```python
from build123d import *

# Parameters (mm, degrees)
F1_DEPTH = 20
F4_W     = 74.543075636
F4_H     = 79.5415919274
F5_DEPTH = 23.0950107676
F7_W     = 62.1554479003
F7_H     = 78.672291711
F8_DEPTH = 25


with BuildPart() as f1:
    # F0 (on Right) → F1 (new body, symmetric)
    with BuildSketch(Plane.YZ):
        Polygon((0, 20), (0, 0), (40, 0), (40, 40), align=None)
    extrude(amount=F1_DEPTH, both=True)

    # F4 (on 3pt) → F5 (cut, through all)
    with BuildSketch(Plane(origin=(6.6666666667, -6.6666666667, 6.6666666667), x_dir=(0.8164965809, 0.4082482905, -0.4082482905), z_dir=(0.5773502692, -0.5773502692, 0.5773502692))):
        with Locations((13.7506006286, 22.7511608973)):
            Rectangle(F4_W, F4_H)
    extrude(amount=F5_DEPTH, mode=Mode.SUBTRACT)

    # F7 (on 3pt) → F8 (cut)
    with BuildSketch(Plane(origin=(-6.6666666667, -6.6666666667, 6.6666666667), x_dir=(0.8164965809, -0.4082482905, 0.4082482905), z_dir=(-0.5773502692, -0.5773502692, 0.5773502692))):
        with Locations((-10.0513882935, 28.4373825416)):
            Rectangle(F7_W, F7_H)
    extrude(amount=F8_DEPTH, mode=Mode.SUBTRACT)


solid = f1.part
```
CAD build for the part. Positions are in the model's coordinates, mm. Round coordinates to 2 decimals unless told otherwise and drop trailing zeros. Order: outer loops, then holes, each group sorted by start corner. A loop starts at its lowest first (then second) coordinate and runs counter-clockwise, first axis right, second up.
Q1. Slice it at A-A (z = 37.5). Write the cut outline in (x, y).
Q2. Drop flat-ended pins along their axis: pin 1 (1 mm diameter, centred on x = 4.5, y = 20, fed in from +Z); pin 2 (1.5 mm diameter, centred on x = -15, y = 6.5, fed in from +Z); pin 3 (4 mm diameter, centred on x = 5, y = 21.5, fed in from +Z). Give the stop position or say it passes through.
Q3. Slice it at B-B (y = 6). Write the cut outline in (x, z), and give its area (3 significant figures).
Q4. Slice it at C-C (x = -8). Write the cut outline in (y, z), and give its area (3 significant figures).
Q5. Slice it at D-D (x = 6.5). Write the cut outline in (y, z), and give its area (3 significant figures).
Q6. Wall check: L1, parallel to Z at x = -13.5, y = 21; L2, parallel to Y at x = 3, z = 35; L3, parallel to Z at x = -15, y = 33.5. Give the ranges that are in metal, low to high.
Results below:
1. outline: (-20, 37.5) - (-17.5, 35) - (17.5, 35) - (20, 37.5) - (20, 40) - (-20, 40) - close
2. pin 1: stops at z = 30.25
2. pin 2: stops at z = 12.56
2. pin 3: stops at z = 31.75
3. outline: (-20, 0) - (20, 0) - (20, 6) - (3, 23) - (-3, 23) - (-20, 6) - close
3. area: 631 mm2
4. outline: (0, 0) - (40, 0) - (40, 40) - (16, 28) - (0, 12) - close
4. area: 1,140 mm2
5. outline: (0, 0) - (40, 0) - (40, 40) - (13, 26.5) - (0, 13.5) - close
5. area: 1,160 mm2
6. L1: z = 0 to 27.5
6. L2: y = 30 to 40
6. L3: z = 0 to 36.75
